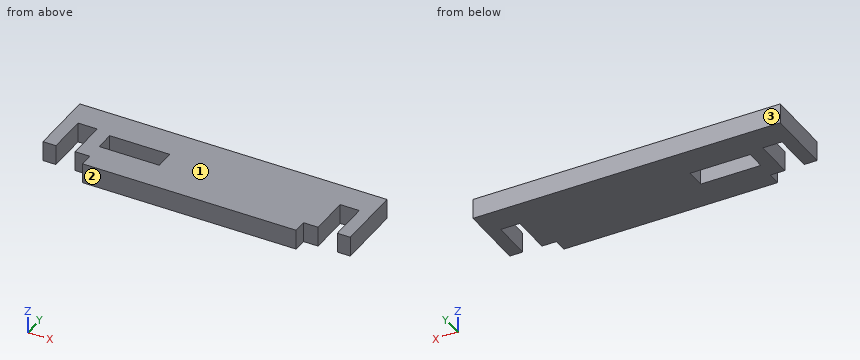
from build123d import *

# Parameters (mm, degrees)
CROQUIS1_W              = 9
CROQUIS1_H              = 2.877
SALIENTE_EXTRUIR1_DEPTH = 3


with BuildPart() as part:
    # Croquis1 → Saliente-Extruir1 (new body)
    with BuildSketch(Plane.XY):
        Polygon((0, 2), (0, 0), (32, 0), (32, 2), (34.1845, 2), (34.1845, 8), (37.0615, 8), (37.0615, 2), (39, 2), (39, 12), (-7, 12), (-7, 2), (-5.0615, 2), (-5.0615, 8), (-2.1845, 8), (-2.1845, 2), align=None)
        with Locations((4.5, 5.9985)):
            Rectangle(CROQUIS1_W, CROQUIS1_H, mode=Mode.SUBTRACT)
    extrude(amount=SALIENTE_EXTRUIR1_DEPTH)


solid = part.part
Here's how the part is built. I have some questions about the finished solid (model axes, mm). Face numbers are marked on the shaded views. Give positions to 0.01 mm unless a question says otherwise; leave off trailing zeros. Order: outer loops, then holes, each group sorted by start corner. A loop starts at its lowest first (then second) coordinate and runs counter-clockwise, first axis right, second up. Notation, with made-up numbers: (19, 38.25) -> (62, 38.25) arc R25 cw to (62, 67.25) -> close; hole circle Ø10 at (53.5, 66). An arc over 180 degrees is marked (long way). One line per item, written item: value. Start each with the question number.
1. We'd pull the mould along Y, two halves only. Please class the marked faces 1, 2 and 3: released by +Y, released by -Y, zero draft, split by the parting line, or undercut.
2. Imagine slicing it at C-C, the plane x = 6. List the corners of the cut face in (y, z) for me.
3. Imagine slicing it at B-B, the plane y = 5.75. List the corners of the cut face in (x, z) for me.
4. Imagine slicing it at A-A, the plane y = 3. List the corners of the cut face in (x, z) for me, plus the area to 3 significant figures.
5. Imagine slicing it at D-D, the plane z = 0.5. List the corners of the cut face in (x, y) for me, plus the area to 3 significant figures.
6. I need wall thicknesses on probe 1 along X at (y, z) = (4.75, 2.8); probe 2 along X at (y, z) = (3.5, 1.4); probe 3 along Y at (x, z) = (4, 0.5). Which ranges of each line are inside material? Lowest first, please. Write a range as from..to.
7. Will these pins go through, and if not, where does the flat tip stop? pin 1 Ø0.9 at (x, z) = (35.5, 1) entering from -Y; pin 2 Ø0.7 at (x, z) = (33, 1) entering from -Y; pin 3 Ø0.6 at (y, z) = (1.5, 1.5) entering from -X.
Values follow:
1. face 1: zero draft
1. face 2: released by -Y
1. face 3: released by +Y
2. outline: (0, 0) -> (4.56, 0) -> (4.56, 3) -> (0, 3) -> close; (7.44, 0) -> (12, 0) -> (12, 3) -> (7.44, 3) -> close
3. outline: (-7, 0) -> (-5.06, 0) -> (-5.06, 3) -> (-7, 3) -> close; (-2.18, 0) -> (0, 0) -> (0, 3) -> (-2.18, 3) -> close; (9, 0) -> (34.18, 0) -> (34.18, 3) -> (9, 3) -> close; (37.06, 0) -> (39, 0) -> (39, 3) -> (37.06, 3) -> close
4. outline: (-7, 0) -> (-5.06, 0) -> (-5.06, 3) -> (-7, 3) -> close; (-2.18, 0) -> (34.18, 0) -> (34.18, 3) -> (-2.18, 3) -> close; (37.06, 0) -> (39, 0) -> (39, 3) -> (37.06, 3) -> close
4. area: 121 mm2
5. outline: (-7, 2) -> (-5.06, 2) -> (-5.06, 8) -> (-2.18, 8) -> (-2.18, 2) -> (0, 2) -> (0, 0) -> (32, 0) -> (32, 2) -> (34.18, 2) -> (34.18, 8) -> (37.06, 8) -> (37.06, 2) -> (39, 2) -> (39, 12) -> (-7, 12) -> close; hole (0, 4.56) -> (9, 4.56) -> (9, 7.44) -> (0, 7.44) -> close
5. area: 464 mm2
6. probe 1: x = -7..-5.06, -2.18..0, 9..34.18, 37.06..39
6. probe 2: x = -7..-5.06, -2.18..34.18, 37.06..39
6. probe 3: y = 0..4.56, 7.44..12
7. pin 1: stops at y = 8
7. pin 2: stops at y = 2
7. pin 3: stops at x = 0
